Geometry check sheet. Reference: the model listing, model coordinates, mm. Face numbers are marked on the shaded views. A direction names the side the tool comes from. Coordinates: 2 decimals unless noted, no trailing zeros. Order: outer loops, then holes, each group sorted by start corner. A loop starts at its lowest first (then second) coordinate and runs counter-clockwise, first axis right, second up. Notation, with made-up numbers: M -16,77 L 16,77 A21 cw 16,113 Z; hole C 27,58 d5. An arc over 180 degrees is marked long. One line per item, written item: value. Start each with the question number.
1) Sectioned sample at C-C, the plane z = 8. Enter the section's corners in (x, y), then the cut area to 3 significant figures.
2) Sectioned sample at D-D, the plane x = -7. Enter the section's corners in (y, z), then the cut area to 3 significant figures.
3) Access from +Z, -Z, +X, -X, +Y, -Y to the whole of each face (thin tool, end or side, straight path). Record for the marked faces 1 and 2.
4) Draft check along X on the marked faces 3, 4 and 5. Enter one of: pulls with the +X half, pulls with the -X half, needs draft (parallel to the pull), parting line crosses it, or undercut.
5) Go/stop test with flat-tipped pins: P1, Ø2.5, axis at x = 8.5, y = -2.5, coming from the +Z side; P2, Ø1, axis at x = -5.5, y = 1, coming from the +Z side; P3, Ø2.5, axis at x = -1.5, y = -1.5, coming from the +Z side. Record where each tip stops, or that it passes through.
6) Sectioned sample at B-B, the plane y = -0.25. Enter the section's corners in (x, z) (3 decimals).
7) Thickness scan on L1, parallel to X at y = -3.25, z = 8.25; L2, parallel to X at y = 3.5, z = 11 (3 decimals); L3, parallel to Z at x = 8, y = 4.25. Record the ranges inside material, lowest first. Write a range as from..to.
8) Sectioned sample at A-A, the plane z = 11.75. Enter the section's corners in (x, y) (3 decimals).
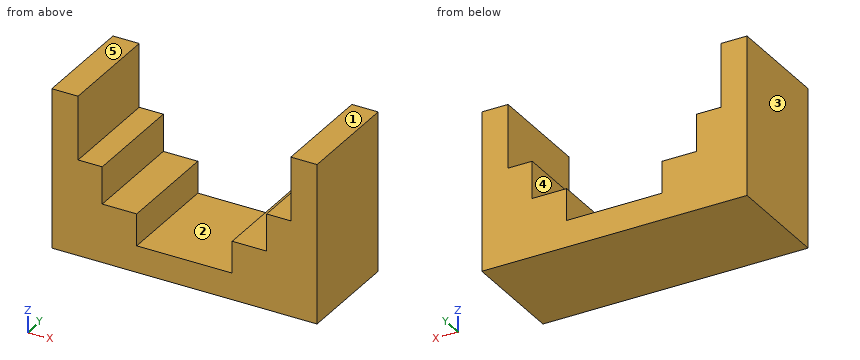
```python
from build123d import *

# Parameters (mm, degrees)
SKETCH1_W           = 25
SKETCH1_H           = 10
BOSS_EXTRUDE1_DEPTH = 15
SKETCH2_W           = 20.05
SKETCH2_H           = 10
CUT_EXTRUDE1_DEPTH  = 6
SKETCH3_W           = 9
SKETCH3_H           = 10
CUT_EXTRUDE2_DEPTH  = 6.5
SKETCH4_W           = 15.5
SKETCH4_H           = 10
CUT_EXTRUDE3_DEPTH  = 3.5


with BuildPart() as part:
    # Sketch1 → Boss-Extrude1 (new body)
    with BuildSketch(Plane.XY):
        Rectangle(SKETCH1_W, SKETCH1_H)
    extrude(amount=BOSS_EXTRUDE1_DEPTH)

    # Sketch2 → Cut-Extrude1 (cut)
    with BuildSketch(Plane.XY.offset(15)):
        Rectangle(SKETCH2_W, SKETCH2_H)
    extrude(amount=-CUT_EXTRUDE1_DEPTH, mode=Mode.SUBTRACT)

    # Sketch3 → Cut-Extrude2 (cut)
    with BuildSketch(Plane.XY.offset(9)):
        Rectangle(SKETCH3_W, SKETCH3_H)
    extrude(amount=-CUT_EXTRUDE2_DEPTH, mode=Mode.SUBTRACT)

    # Sketch4 → Cut-Extrude3 (cut)
    with BuildSketch(Plane.XY.offset(9)):
        Rectangle(SKETCH4_W, SKETCH4_H)
    extrude(amount=-CUT_EXTRUDE3_DEPTH, mode=Mode.SUBTRACT)


solid = part.part
```
Final values:
1. outline: M -12.5,-5 L -7.75,-5 L -7.75,5 L -12.5,5 Z; M 7.75,-5 L 12.5,-5 L 12.5,5 L 7.75,5 Z
1. area: 95.0 mm^2
2. outline: M -5,0 L 5,0 L 5,5.5 L -5,5.5 Z
2. area: 55.0 mm^2
3. face 1: +Z, +X, -X, +Y, -Y
3. face 2: +Z, +Y, -Y
4. face 3: pulls with the -X half
4. face 4: undercut
4. face 5: needs draft
5. P1: stops at z = 9
5. P2: stops at z = 5.5
5. P3: stops at z = 2.5
6. outline: M -12.5,0 L 12.5,0 L 12.5,15 L 10.025,15 L 10.025,9 L 7.75,9 L 7.75,5.5 L 4.5,5.5 L 4.5,2.5 L -4.5,2.5 L -4.5,5.5 L -7.75,5.5 L -7.75,9 L -10.025,9 L -10.025,15 L -12.5,15 Z
7. L1: x = -12.5..-7.75, 7.75..12.5
7. L2: x = -12.5..-10.025, 10.025..12.5
7. L3: z = 0..9
8. outline: M -12.5,-5 L -10.025,-5 L -10.025,5 L -12.5,5 Z; M 10.025,-5 L 12.5,-5 L 12.5,5 L 10.025,5 Z
